Design review of the part built by this model. Coordinates are the model's own, in mm. A direction names the side the tool comes from. Coordinates: 2 decimals unless noted, no trailing zeros. Loops run counter-clockwise (first coordinate to the right, second up) from the corner with the lowest first, then second, coordinate; pieces in that order, holes last. Notation, with made-up numbers: M 55,28.25 L 74,28.25 A13 ccw 74,32.25 Z; hole C -16.75,30.25 d7. An arc over 180 degrees is marked long. One line per item, written item: value.
```python
from build123d import *

# Parameters (mm, degrees)
SKETCH1_W           = 98
SKETCH1_H           = 54
SKETCH1_R           = 8
SKETCH1_R_2         = 5.25
SKETCH1_R_3         = 2.25
BOSS_EXTRUDE1_DEPTH = 49
FILLET1_R           = 10
SKETCH2_R           = 1.810942065
CUT_EXTRUDE1_DEPTH  = 145.300803777
SKETCH3_W           = 80.000000001
SKETCH3_H           = 24.290118096
CUT_EXTRUDE2_DEPTH  = 145.300803849


with BuildPart() as part:
    # Sketch1 → Boss-Extrude1 (new body)
    with BuildSketch(Plane.XY):
        with Locations((-75.521973847, 14.434233909)):
            Rectangle(SKETCH1_W, SKETCH1_H)
        with Locations((-97.771973847, 12.934233909)):
            Circle(SKETCH1_R, mode=Mode.SUBTRACT)
        with Locations((-108.771973847, 30.434233909)):
            Circle(SKETCH1_R_2, mode=Mode.SUBTRACT)
        with Locations((-98.271973847, -6.565766091)):
            Circle(SKETCH1_R_2, mode=Mode.SUBTRACT)
        with Locations((-62.771973847, 30.434233909)):
            Circle(SKETCH1_R_2, mode=Mode.SUBTRACT)
        with BuildLine():
            ThreePointArc((-78.528692534, 21.62979932), (-88.924408217, 33.051798322), (-85.70721761, 17.946082504))
            ThreePointArc((-85.70721761, 17.946082504), (-68.673659404, -6.411199365), (-78.528692534, 21.62979932))
        make_face(mode=Mode.SUBTRACT)
        with Locations((-62.771973847, 30.434233909)):
            Circle(SKETCH1_R_2)
        with Locations((-62.771973847, 30.434233909)):
            Circle(SKETCH1_R_3, mode=Mode.SUBTRACT)
        with Locations((-108.771973847, 30.434233909)):
            Circle(SKETCH1_R_2)
        with Locations((-108.771973847, 30.434233909)):
            Circle(SKETCH1_R_3, mode=Mode.SUBTRACT)
    extrude(amount=BOSS_EXTRUDE1_DEPTH)

    # Fillet1
    fillet1_edges = [part.edges().sort_by_distance(p)[0] for p in [
        (-124.521973847, 14.434233909, 0),
        (-26.521973847, 14.434233909, 0),
    ]]
    fillet(fillet1_edges, radius=FILLET1_R)

    # Sketch2 → Cut-Extrude1 (cut, through all)
    with BuildSketch(Plane(origin=(0, 41.434233909, 0), x_dir=(1, 0, 0), z_dir=(0, 1, 0))):
        with Locations(Location((-50.601973847, -39, 0), (0, 0, 270))):
            Circle(SKETCH2_R)
        with Locations(Location((-100.441973847, -39, 0), (0, 0, 270))):
            Circle(SKETCH2_R)
    extrude(amount=-CUT_EXTRUDE1_DEPTH, mode=Mode.SUBTRACT)

    # Sketch3 → Cut-Extrude2 (cut, through all)
    with BuildSketch(Plane.XZ.offset(12.565766091)):
        with Locations((-75.521627845, 36.854940952)):
            Rectangle(SKETCH3_W, SKETCH3_H)
    extrude(amount=-CUT_EXTRUDE2_DEPTH, mode=Mode.SUBTRACT)


solid = part.part
```
(1) To check wall thickness, follow line 1 along X through (y, z) = (23.5, 25); line 2 along X through (y, z) = (15, 21.5); line 3 along X through (y, z) = (17, 5.5). State the ranges of each line that lie inside material, in increasing order. Write a range as [from, to].
Reply:
line 1: x = [-124.52, -115.52], [-35.52, -26.52]
line 2: x = [-124.52, -105.5], [-90.04, -88.17], [-62.88, -26.52]
line 3: x = [-123.45, -104.66], [-90.88, -86.64], [-64.4, -27.59]
(2) Insertion check: pin 1 (2 mm diameter, centred on x = -52.5, y = 20, fed in from +Z). The pin has a flat end and moves straight along its axis. Give the tip position at first contact, or say it passes through.
Reply:
pin 1: stops at z = 24.71
(3) We need section B-B on y = 1. State the section outline as (x, z) points.
Reply:
outline: M -124.52,10 A10 ccw -114.52,0 L -89.3,0 L -89.3,24.71 L -115.52,24.71 L -115.52,49 L -124.52,49 Z; M -61.75,0 L -36.52,0 A10 ccw -26.52,10 L -26.52,49 L -35.52,49 L -35.52,24.71 L -61.75,24.71 Z
(4) Mouldability with a two-part tool opening along X and no side actions: class faces 3 (the flat face through (-31, 15, 49)), 4 (the cylindrical face through (-121.67, 14.812, 3.007)), 5 (the cylindrical face through (-69.215, -6.675, 12.182)) as released by +X, released by -X, zero draft, split by the parting line, or undercut.
Reply:
face 3: zero draft
face 4: released by -X
face 5: undercut
(5) Tool access review of faces 1 (the cylindrical face through (-93.264, -4.989, 12.182)), 2 (the flat face through (-35.522, 14, 37)): name each direction out of +Z, -Z, +X, -X, +Y, -Y from which nothing blocks a thin tool from reaching the whole face with its end or side.
Reply:
face 1: +Z, -Z
face 2: +Z, +Y, -Y
(6) We need section C-C on x = -80. State the section outline as (y, z) points, then the cut area to 3 significant figures.
Reply:
outline: M -12.57,0 L -7.38,0 L -7.38,24.71 L -12.57,24.71 Z; M 31.95,0 L 41.43,0 L 41.43,24.71 L 31.95,24.71 Z
area: 362 mm2
(7) We need section D-D on y = 10.5. State the section outline as (x, z) points, then the cut area to 3 significant figures.
Reply:
outline: M -124.52,10 A10 ccw -114.52,0 L -105.39,0 L -105.39,24.71 L -115.52,24.71 L -115.52,49 L -124.52,49 Z; M -90.15,0 L -90.09,0 L -90.09,24.71 L -90.15,24.71 Z; M -60.95,0 L -36.52,0 A10 ccw -26.52,10 L -26.52,49 L -35.52,49 L -35.52,24.71 L -60.95,24.71 Z
area: 1,720 mm2
(8) We need section A-A on z = 36.5. State the section outline as (x, y) points.
Reply:
outline: M -124.52,-12.57 L -115.52,-12.57 L -115.52,41.43 L -124.52,41.43 Z; M -35.52,-12.57 L -26.52,-12.57 L -26.52,41.43 L -35.52,41.43 Z
